```python
from build123d import *

# Parameters (mm, degrees)
ESQUISSE4_W             = 12
ESQUISSE4_H             = 2
ESQUISSE4_W_2           = 37.75
BOSS_EXTRU_2_DEPTH      = 20
ESQUISSE5_R             = 1.75
ENL_V_MAT_EXTRU_1_DEPTH = 57.846833685


with BuildPart() as part:
    # Esquisse4 → Boss.-Extru.2 (new body)
    with BuildSketch(Plane.XY):
        with Locations((-46.75, -4)):
            Rectangle(ESQUISSE4_W, ESQUISSE4_H)
        Polygon((-40.75, -3), (-37.75, 0), (-37.75, 2), (-42.75, -3), align=None)
        with Locations((-18.875, 1)):
            Rectangle(ESQUISSE4_W_2, ESQUISSE4_H)
        with Locations((18.875, 1)):
            Rectangle(ESQUISSE4_W_2, ESQUISSE4_H)
        Polygon((37.75, 2), (37.75, 0), (40.75, -3), (42.75, -3), align=None)
        with Locations((46.75, -4)):
            Rectangle(ESQUISSE4_W, ESQUISSE4_H)
    extrude(amount=BOSS_EXTRU_2_DEPTH)

    # Esquisse5 → Enlèv. mat.-Extru.1 (cut, through all)
    with BuildSketch(Plane(origin=(0, 2, 0), x_dir=(1, 0, 0), z_dir=(0, 1, 0))):
        with Locations(Location((-46.25, -15.5, 0), (0, 0, 270))):
            Circle(ESQUISSE5_R)
        with Locations(Location((46.25, -15.5, 0), (0, 0, 270))):
            Circle(ESQUISSE5_R)
    extrude(amount=-ENL_V_MAT_EXTRU_1_DEPTH, mode=Mode.SUBTRACT)


solid = part.part
```
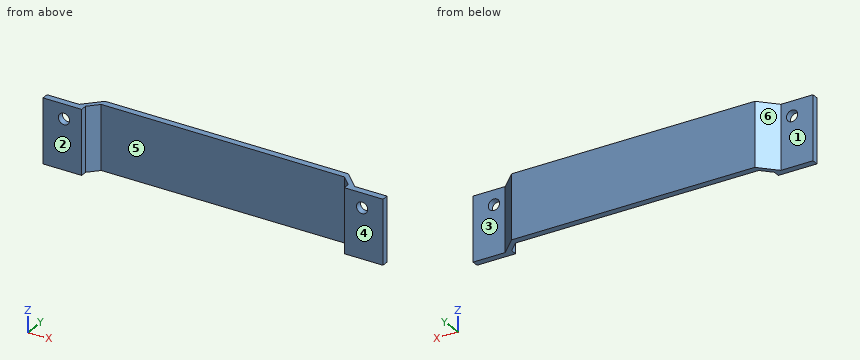
Geometry check sheet. Reference: the model listing, model coordinates, mm. Face numbers are marked on the shaded views. A direction names the side the tool comes from. Coordinates: 2 decimals unless noted, no trailing zeros. Order: outer loops, then holes, each group sorted by start corner. A loop starts at its lowest first (then second) coordinate and runs counter-clockwise, first axis right, second up. Notation, with made-up numbers: (23, -10.75) - (63, -10.75) arc R29 cw to (63, 20.25) - close; hole circle Ø3 at (68.5, 74). An arc over 180 degrees is marked (long way). Answer as a JSON object with one key per item and string values. Group by question number.
Item 1: Tool access check on the marked faces 1, 2 and 3. Record the directions out of +Z, -Z, +X, -X, +Y, -Y that give a thin tool (end or side, any length) a straight path to the whole face; none if there is none.
Item 2: Draft check along X on the marked faces 4, 5 and 6. Enter one of: +X half, -X half, draft (parallel to the pull), parting line (faces both ways), or undercut.
Item 3: Scan lines: probe 1 along X at (y, z) = (-4.3, 15.5); probe 2 along Y at (x, z) = (11, 6.5); probe 3 along X at (y, z) = (-0.25, 13). Record each from-to range of solid material in increasing order.
Item 4: Sectioned sample at D-D, the plane y = 1. Record the cut outline in (x, z).
Item 5: Depth check by flat-ended pin: pin 1 Ø5.5 at (x, z) = (-46.25, 15.5) entering from +Y; pin 2 Ø12 at (x, z) = (-33.5, 9) entering from -Y; pin 3 Ø3 at (x, z) = (46.25, 15.5) entering from +Y; pin 4 Ø10 at (x, z) = (-6.5, 10) entering from -Y. Enter the tip coordinate at first touch or a pass-through.
Item 6: Sectioned sample at A-A, the plane z = 15.5. Record the cut outline in (x, y), and give its area (3 significant figures).
Item 7: Sectioned sample at C-C, the plane z = 6.75. Record the cut outline in (x, y), and give its area (3 significant figures).
Item 8: Sectioned sample at B-B, the plane x = 46.25. Record the cut outline in (y, z), and give its area (3 significant figures).
Resolved:
{
 "1": {"face 1": "+Z, -Z, -X, +Y", "face 2": "+Z, -Z, +X, -X, -Y", "face 3": "+Z, -Z, +X, +Y"},
 "2": {"face 4": "draft", "face 5": "undercut", "face 6": "-X half"},
 "3": {"probe 1": "-52.75 to -48, -44.5 to -40.75, 40.75 to 44.5, 48 to 52.75", "probe 2": "0 to 2", "probe 3": "-40 to -38, 38 to 40"},
 "4": {"outline": "(-38.75, 0) - (38.75, 0) - (38.75, 20) - (-38.75, 20) - close"},
 "5": {"pin 1": "y = -3", "pin 2": "y = -1.75", "pin 3": "through", "pin 4": "y = 0"},
 "6": {"outline": "(-52.75, -5) - (-48, -5) - (-48, -3) - (-52.75, -3) - close; (-44.5, -5) - (-40.75, -5) - (-40.75, -3) - (-37.75, 0) - (37.75, 0) - (40.75, -3) - (40.75, -5) - (44.5, -5) - (44.5, -3) - (42.75, -3) - (37.75, 2) - (-37.75, 2) - (-42.75, -3) - (-44.5, -3) - close; (48, -5) - (52.75, -5) - (52.75, -3) - (48, -3) - close", "area": "201 mm^2"},
 "7": {"outline": "(-52.75, -5) - (-40.75, -5) - (-40.75, -3) - (-37.75, 0) - (37.75, 0) - (40.75, -3) - (40.75, -5) - (52.75, -5) - (52.75, -3) - (42.75, -3) - (37.75, 2) - (-37.75, 2) - (-42.75, -3) - (-52.75, -3) - close", "area": "215 mm^2"},
 "8": {"outline": "(-5, 0) - (-3, 0) - (-3, 13.75) - (-5, 13.75) - close; (-5, 17.25) - (-3, 17.25) - (-3, 20) - (-5, 20) - close", "area": "33.0 mm^2"}
}
